Geometry: see drawing. Coordinates: mm, zero at the bounding-box minimum. A direction names the side the tool comes from. Give positions to 0.01 mm unless a question says otherwise; leave off trailing zeros. Order: outer loops, then holes, each group sorted by start corner. A loop starts at its lowest first (then second) coordinate and runs counter-clockwise, first axis right, second up. Notation, with made-up numbers: (50, -20) - (65, -20) arc R4 ccw to (65, -15) - close; hole circle Ø7 at (40, 2). An arc over 180 degrees is marked (long way). Put each result on its own line as item: value. Start each with the question number.
1. Section A-A on z = 20. Return the cut outline in (x, y), plus the area to 3 significant figures.
2. Ray query, line 1 along X through (y, z) = (19, 19.5); line 2 along Y through (x, z) = (24, 28.5); line 3 along X through (y, z) = (50, 29). Return the intervals inside material, ascending. Write a range as from..to.
3. Mould query, pull axis X, two halves, no side actions, for the marked faces 5, 6 and 7. Classes: pulls with the +X half, pulls with the -X half, needs draft (parallel to the pull), parting line crosses it, or undercut.
4. Set-up query: the marked faces 1, 2, 3 and 4. Return all of +Z, -Z, +X, -X, +Y, -Y with unobstructed straight access to the full face (end or side cutting, diameter ignored); none if empty.
5. Section D-D on y = 53. Return the cut outline in (x, z), plus the area to 3 significant figures.
6. Section C-C on x = 42. Return the cut outline in (y, z), plus the area to 3 significant figures.
7. Section B-B on y = 9.5. Return the cut outline in (x, z).
8. First-contact query: P1, Ø4, axis at x = 16.5, z = 20.5, coming from the -Y side; P2, Ø3, axis at x = 84, z = 6.5, coming from the +Y side; P3, Ø3.5, axis at x = 152, y = 10.5, coming from the -Z side. Flat tips, straight axial feed; report the tip coordinate or a pass-through.
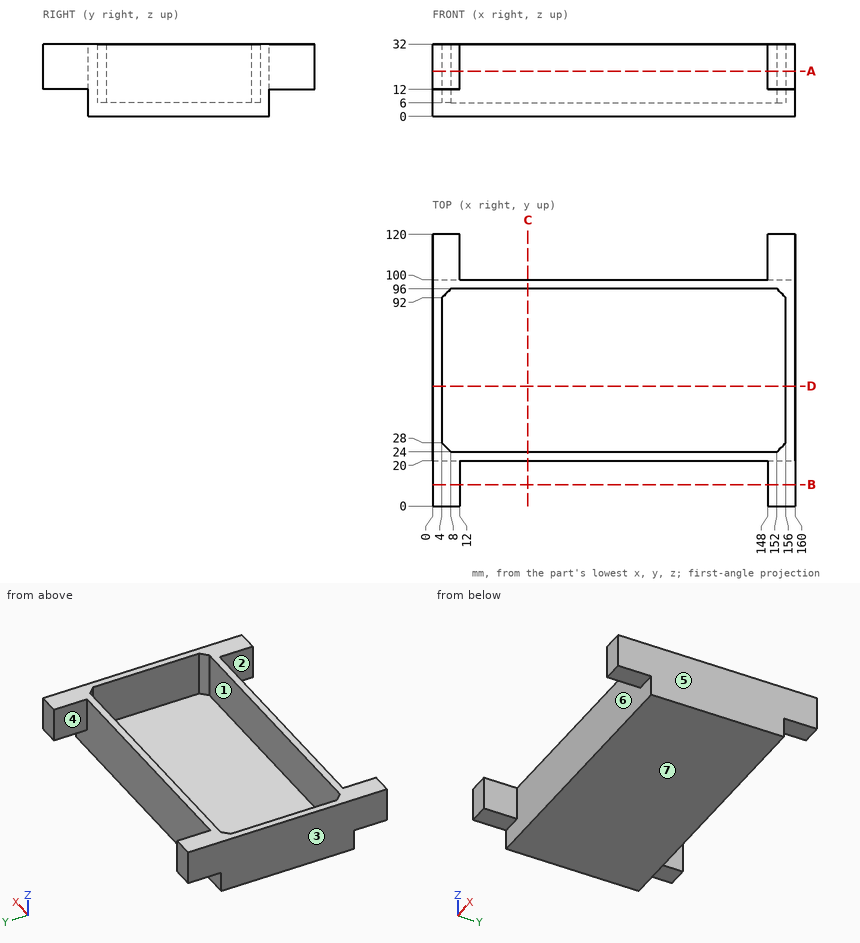
Resolved:
1. outline: (0, 0) - (12, 0) - (12, 20) - (148, 20) - (148, 0) - (160, 0) - (160, 120) - (148, 120) - (148, 100) - (12, 100) - (12, 120) - (0, 120) - close; hole (4, 28) - (8, 24) - (152, 24) - (156, 28) - (156, 92) - (152, 96) - (8, 96) - (4, 92) - close
1. area: 2,850 mm^2
2. line 1: 0..12, 148..160
2. line 2: 20..24, 96..100
2. line 3: 0..4, 156..160
3. face 5: pulls with the +X half
3. face 6: undercut
3. face 7: needs draft
4. face 1: +Z
4. face 2: +Z, -Z, -Y
4. face 3: +Z, -Z, -X, +Y, -Y
4. face 4: +Z, -Z, +Y
5. outline: (0, 0) - (160, 0) - (160, 32) - (156, 32) - (156, 6) - (4, 6) - (4, 32) - (0, 32) - close
5. area: 1,170 mm^2
6. outline: (20, 0) - (100, 0) - (100, 32) - (96, 32) - (96, 6) - (24, 6) - (24, 32) - (20, 32) - close
6. area: 688 mm^2
7. outline: (0, 12) - (12, 12) - (12, 32) - (0, 32) - close; (148, 12) - (160, 12) - (160, 32) - (148, 32) - close
8. P1: y = 20
8. P2: y = 100
8. P3: z = 12
